Work out the finished part from the listing and answer in its coordinate system (mm). A direction names the side the tool comes from. Round coordinates to 2 decimals unless told otherwise and drop trailing zeros. Loops run counter-clockwise (first coordinate to the right, second up) from the corner with the lowest first, then second, coordinate; pieces in that order, holes last. Notation, with made-up numbers: (-5.75, -14.5) - (2.25, -14.5) arc R13 ccw to (2.25, 8.5) - close; hole circle Ø4 at (11, 2.5). An arc over 180 degrees is marked (long way). Return JSON: item names as keys, results as strings.
from build123d import *

# Parameters (mm, degrees)
SKETCH1_W           = 42
SKETCH1_H           = 40
SKETCH1_R           = 3
SKETCH1_R_2         = 2.5
BOSS_EXTRUDE1_DEPTH = 5
FILLET1_R           = 5
SKETCH2_R           = 3
BOSS_EXTRUDE2_DEPTH = 25
FILLET2_R           = 2


with BuildPart() as part:
    # Sketch1 → Boss-Extrude1 (new body)
    with BuildSketch(Plane.XY):
        Rectangle(SKETCH1_W, SKETCH1_H)
        Circle(SKETCH1_R, mode=Mode.SUBTRACT)
        with Locations((-15, 15)):
            Circle(SKETCH1_R_2, mode=Mode.SUBTRACT)
        with Locations((15, 15)):
            Circle(SKETCH1_R_2, mode=Mode.SUBTRACT)
        with Locations(Location((15, -15, 0), (0, 0, 180))):
            Circle(SKETCH1_R_2, mode=Mode.SUBTRACT)
        with Locations(Location((-15, -15, 0), (0, 0, 180))):
            Circle(SKETCH1_R_2, mode=Mode.SUBTRACT)
    extrude(amount=BOSS_EXTRUDE1_DEPTH)

    # Fillet1
    fillet1_edges = [part.edges().sort_by_distance(p)[0] for p in [
        (21, -20, 2.5),
        (-21, -20, 2.5),
        (-21, 20, 2.5),
        (21, 20, 2.5),
    ]]
    fillet(fillet1_edges, radius=FILLET1_R)

    # Sketch2 → Boss-Extrude2 (add)
    with BuildSketch(Plane.XY.offset(5)):
        with BuildLine():
            ThreePointArc((-15.71875, -2.98678731), (0, -16), (15.71875, -2.98678731))
            ThreePointArc((15.71875, -2.98678731), (13, 0), (15.71875, 2.98678731))
            ThreePointArc((15.71875, 2.98678731), (0, 16), (-15.71875, 2.98678731))
            ThreePointArc((-15.71875, 2.98678731), (-13, 0), (-15.71875, -2.98678731))
        make_face()
        Circle(SKETCH2_R, mode=Mode.SUBTRACT)
    extrude(amount=BOSS_EXTRUDE2_DEPTH)

    # Fillet2
    fillet2_edges = [part.edges().sort_by_distance(p)[0] for p in [
        (15.71875, -2.98678731, 17.5),
        (15.71875, 2.98678731, 17.5),
        (-15.71875, 2.98678731, 17.5),
        (-15.71875, -2.98678731, 17.5),
    ]]
    fillet(fillet2_edges, radius=FILLET2_R)


solid = part.part
1) Section A-A (y = 0) is taken. Give the vertices of the cut face in (x, z), and give its area (3 significant figures).
Verdict:
{"outline": "(-21, 0) - (-3, 0) - (-3, 30) - (-13, 30) - (-13, 5) - (-21, 5) - close; (3, 0) - (21, 0) - (21, 5) - (13, 5) - (13, 30) - (3, 30) - close", "area": "680 mm2"}
2) Section B-B (x = 0) is taken. Give the vertices of the cut face in (y, z).
Verdict:
{"outline": "(-20, 0) - (-3, 0) - (-3, 30) - (-16, 30) - (-16, 5) - (-20, 5) - close; (3, 0) - (20, 0) - (20, 5) - (16, 5) - (16, 30) - (3, 30) - close"}
3) Determine the mould class of faces 5 (the flat face through (0, 20, 2)), 6 (the cylindrical face through (17, -13.5, 2.5)), 7 (the cylindrical face through (19, -19, 3)) for opening direction Y: pulls with the +Y half, pulls with the -Y half, needs draft (parallel to the pull), parting line crosses it, or undercut.
Verdict:
{"face 5": "pulls with the +Y half", "face 6": "undercut", "face 7": "pulls with the -Y half"}
4) Flat-ended cylindrical pins translate along their axes: pin 1 (4.5 mm diameter, centred on x = 15, y = -15, fed in from +Z); pin 2 (6 mm diameter, centred on y = 16, z = 4.5, fed in from -X); pin 3 (12 mm diameter, centred on y = 16, z = 18, fed in from -X); pin 4 (6.5 mm diameter, centred on x = -15, y = 15, fed in from +Z). Find the tip coordinate at first contact, or state that the pin passes through.
Verdict:
{"pin 1": "passes through", "pin 2": "stops at x = -21", "pin 3": "stops at x = -12.49", "pin 4": "stops at z = 5"}
5) A tool of negligible diameter and unlimited length cuts with its end or side. For faces 1 (the cylindrical face through (-13, 0, 17)), 2 (the flat face through (-14, 0, 5)), 3 (the cylindrical face through (0, 16, 17)), 4 (the cylindrical face through (13, 0, 17)), from which of +Z, -Z, +X, -X, +Y, -Y can it reach the whole face along a straight path? Write none if from no direction.
Verdict:
{"face 1": "+Z, -X", "face 2": "+Z", "face 3": "+Z, +Y", "face 4": "+Z, +X"}
6) Section C-C (y = -8) is taken. Give the vertices of the cut face in (x, z).
Verdict:
{"outline": "(-21, 0) - (21, 0) - (21, 5) - (13.86, 5) - (13.86, 30) - (-13.86, 30) - (-13.86, 5) - (-21, 5) - close"}
7) Section D-D (x = 8) is taken. Give the vertices of the cut face in (y, z).
Verdict:
{"outline": "(-20, 0) - (20, 0) - (20, 5) - (13.86, 5) - (13.86, 30) - (-13.86, 30) - (-13.86, 5) - (-20, 5) - close"}
8) Find the intervals of material crossed by L1, parallel to Y at x = 15, z = 3; L2, parallel to X at y = -15, z = 2.45; L3, parallel to Z at x = -17, y = -1.5, in increasing order.
Verdict:
{"L1": "y = -20 to -17.5, -12.5 to 12.5, 17.5 to 20", "L2": "x = -21 to -17.5, -12.5 to 12.5, 17.5 to 21", "L3": "z = 0 to 5"}
